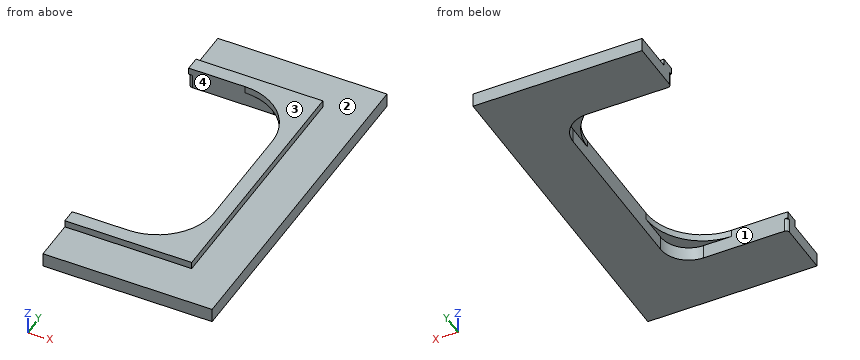
Autodesk Inventor part; units mm, degrees
ref_plane "YZ Plane" through (0, 0, 0) normal (1, 0, 0) x (0, 1, 0)
ref_plane "XZ Plane" through (0, 0, 0) normal (0, 1, 0) x (-1, 0, 0)
ref_plane "XY Plane" through (0, 0, 0) normal (0, 0, 1) x (1, 0, 0)
sketch "Sketch1" plane through (0, 0, 0) normal (0, 0, 1) x (1, 0, 0)
  line L0 (0, 0) -> (76.2, 0)
  line L1 (76.2, 0) -> (76.2, 152.4)
  line L2 (76.2, 152.4) -> (0, 152.4)
  line L3 (0, 152.4) -> (0, 0)
  line L4 (0, 127) -> (50.8, 127)
  line L5 (50.8, 127) -> (50.8, 25.4)
  line L6 (50.8, 25.4) -> (0, 25.4)
  line L7 (0, 25.4) -> (0, 127)
  point P0 (0, 25.4)
  point P1 (76.2, 76.2)
  dimension "d0" = 101.6
  dimension "d1" = 50.8
  dimension "d2" = 25.4
  dimension "d4" = 25.4
  dimension "d9" = 25.4
extrude "Extrusion1" add sketch "Sketch1" along normal blind 6.35 contours L3 L6 L5 L4 L2 L1 L0
fillet "Fillet1" radius 12.7 2 edges at (50.8, 127, 3.175) (50.8, 25.4, 3.175)
fillet "Fillet2" radius 1.5875 2 edges at (0, 127, 3.175) (0, 25.4, 3.175)
sketch "Sketch2" plane through (0, 0, 6.35) normal (0, 0, 1) x (1, 0, 0)
  line L0 (0, 127) -> (25.4, 127)
  line L1 (50.8, 101.6) -> (50.8, 50.8)
  line L2 (25.4, 25.4) -> (19.0762, 25.4)
  line L3 (1.5875, 127) -> (38.1, 127)
  arc A0 (50.8, 101.6) -> (25.4, 127) centre (25.4, 101.6) ccw
  arc A1 (25.4, 25.4) -> (50.8, 50.8) centre (25.4, 50.8) ccw
  line L4 (38.1, 25.4) -> (1.5875, 25.4)
  line L5 (76.2, 0) -> (76.2, 152.4)
  line L6 (0, 127) -> (0, 133.35)
  line L7 (0, 133.35) -> (57.15, 133.35)
  line L8 (57.15, 133.35) -> (57.15, 19.05)
  line L9 (57.15, 19.05) -> (0, 19.05)
  line L10 (0, 19.05) -> (0, 25.4)
  line L11 (0, 25.4) -> (1.5875, 25.4)
  line L12 (0, 152.4) -> (0, 128.5875)
  line L13 (0, 23.8125) -> (0, 0)
  point P0 (0.7937, 25.4)
  dimension "d11" = 25.4
  dimension "d12" = 25.4
  dimension "d13" = 25.4
  dimension "d14" = 6.35
  dimension "d15" = 6.35
  dimension "d16" = 6.35
extrude "Extrusion2" add sketch "Sketch2" along normal blind 3.175
equation "\"d15\" = d14"
equation "\"d16\" = d14"
properties part number "ChassisInterfaceFix"
Source: CAD feature listing. Evaluate the final solid. Frame: model axes, mm. Face numbers are marked on the shaded views. A direction names the side the tool comes from. Give positions to 0.01 mm unless a question says otherwise; leave off trailing zeros. Order: outer loops, then holes, each group sorted by start corner. A loop starts at its lowest first (then second) coordinate and runs counter-clockwise, first axis right, second up. Notation, with made-up numbers: (11.5, 83.5) -> (30.5, 83.5) arc R22 cw to (30.5, 95.5) -> close; hole circle Ø8 at (7, 56). An arc over 180 degrees is marked (long way). Use a Markdown table: item, result.
Q1. Section D-D (x = 54.5). Return the cut outline in (y, z) (3 decimals), and give its area (3 significant figures).
A:
| item | result |
|---|---|
| outline | (0, 0) -> (152.4, 0) -> (152.4, 6.35) -> (133.35, 6.35) -> (133.35, 9.525) -> (19.05, 9.525) -> (19.05, 6.35) -> (0, 6.35) -> close |
| area | 1,330 mm^2 |
Q2. First-contact query: P1, Ø12.5, axis at x = 40, y = 41, coming from the -Z side; P2, Ø3, axis at y = 72.5, z = 6.5, coming from the -X side; P3, Ø1.6, axis at x = 21.5, z = 8.5, coming from the +Y side. Flat tips, straight axial feed; report the tip coordinate or a pass-through.
A:
| item | result |
|---|---|
| P1 | through |
| P2 | x = 50.8 |
| P3 | y = 133.35 |
Q3. Material intervals for line 1 (Y direction, x = 3, z = 1.75); line 2 (X direction, y = 96, z = 8); line 3 (Y direction, x = 25, z = 7), sorted ascending. Write a range as [from, to].
A:
| item | result |
|---|---|
| line 1 | [0, 25.4], [127, 152.4] |
| line 2 | [50.8, 57.15] |
| line 3 | [19.05, 25.4], [127, 133.35] |
Q4. Section C-C (y = 131). Return the cut outline in (x, z) (3 decimals), and give its area (3 significant figures).
A:
| item | result |
|---|---|
| outline | (0, 0) -> (76.2, 0) -> (76.2, 6.35) -> (57.15, 6.35) -> (57.15, 9.525) -> (0, 9.525) -> close |
| area | 665 mm^2 |
Q5. Section A-A (x = 23). Return the cut outline in (y, z) (3 decimals), and give its area (3 significant figures).
A:
| item | result |
|---|---|
| outline | (0, 0) -> (25.4, 0) -> (25.4, 9.525) -> (19.05, 9.525) -> (19.05, 6.35) -> (0, 6.35) -> close; (127, 0) -> (152.4, 0) -> (152.4, 6.35) -> (133.35, 6.35) -> (133.35, 9.525) -> (127, 9.525) -> close |
| area | 363 mm^2 |
Q6. Access query for the marked faces 3 and 4. Directions: +Z, -Z, +X, -X, +Y, -Y. A direction counts if a zero-diameter tool reaches every point of the face in a straight line with its end or side. Return the directions, or none.
A:
| item | result |
|---|---|
| face 3 | +Z, +X, -X, +Y, -Y |
| face 4 | -Z, -X |
Q7. Section B-B (z = 8). Return the cut outline in (x, y), and give its area (3 significant figures).
A:
| item | result |
|---|---|
| outline | (0, 19.05) -> (57.15, 19.05) -> (57.15, 133.35) -> (0, 133.35) -> (0, 127) -> (25.4, 127) arc R25.4 cw to (50.8, 101.6) -> (50.8, 50.8) arc R25.4 cw to (25.4, 25.4) -> (0, 25.4) -> close |
| area | 1,650 mm^2 |
Q8. Pull-direction query (Y, two-part tool) for the marked faces 1 and 2; classes: +Y half, -Y half, draft (parallel to the pull), parting line (faces both ways), or undercut.
A:
| item | result |
|---|---|
| face 1 | undercut |
| face 2 | draft |
